Design review of the part built by this model. Coordinates are the model's own, in mm. Face numbers are marked on the shaded views. A direction names the side the tool comes from. Round coordinates to 2 decimals unless told otherwise and drop trailing zeros. Loops run counter-clockwise (first coordinate to the right, second up) from the corner with the lowest first, then second, coordinate; pieces in that order, holes last. Notation, with made-up numbers: (78, 7) -> (115, 7) arc R34 ccw to (115, 37) -> close; hole circle Ø6 at (38.5, 53.5). An arc over 180 degrees is marked (long way). Write each question's results on one line, items separated by ' | '. Start each with the question number.
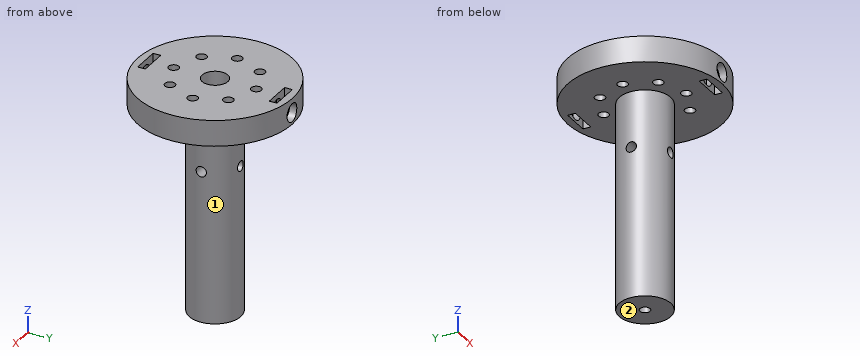
from build123d import *

# Parameters (mm, degrees)
SKETCH1_R               = 30
BOSS_EXTRUDE1_DEPTH     = 10
SKETCH2_R               = 10
BOSS_EXTRUDE2_DEPTH     = 80
SKETCH2_2_R             = 10
BOSS_EXTRUDE3_DEPTH     = 20
SKETCH5_R               = 5
CUT_EXTRUDE1_DEPTH      = 100.498743711
SKETCH6_R               = 2
CUT_EXTRUDE2_DEPTH      = 91.553851381
CIRPATTERN1_COUNT       = 2
CIRPATTERN1_ANGLE       = 90
CUT_EXTRUDE3_DEPTH      = 100.498743801
CUT_EXTRUDE3_DEPTH_BACK = 100.498743801
SKETCH7_R               = 2
SKETCH9_W               = 11
SKETCH9_H               = 3
CUT_EXTRUDE5_DEPTH      = 10
SKETCH10_R              = 3.5
CUT_EXTRUDE6_DEPTH      = 8
SKETCH17_R              = 7.355644599
BOSS_EXTRUDE4_DEPTH     = 25
SKETCH18_R              = 2
CUT_EXTRUDE7_DEPTH      = 10


with BuildPart() as part:
    # Sketch1 → Boss-Extrude1 (new body)
    with BuildSketch(Plane.XY):
        Circle(SKETCH1_R)
    extrude(amount=BOSS_EXTRUDE1_DEPTH)

    # Sketch2 → Boss-Extrude2 (add)
    with BuildSketch(Plane(origin=(0, 0, 0), x_dir=(-1, 0, 0), z_dir=(0, 0, -1))):
        Circle(SKETCH2_R)
    extrude(amount=BOSS_EXTRUDE2_DEPTH)

    # Sketch2_2 → Boss-Extrude3 (add)
    with BuildSketch(Plane(origin=(0, 0, 0), x_dir=(-1, 0, 0), z_dir=(0, 0, -1))):
        Circle(SKETCH2_2_R)
    extrude(amount=BOSS_EXTRUDE3_DEPTH)

    # Sketch5 → Cut-Extrude1 (cut, through all)
    with BuildSketch(Plane(origin=(0, 0, -80), x_dir=(-1, 0, 0), z_dir=(0, 0, -1))):
        Circle(SKETCH5_R)
    extrude(amount=-CUT_EXTRUDE1_DEPTH, mode=Mode.SUBTRACT)

    # Sketch6 → Cut-Extrude2 (cut, symmetric)
    with BuildSketch(Plane(origin=(0, 0, 0), x_dir=(1, 0, 0), z_dir=(0, 1, 0))):
        with Locations(Location((0, 21.5, 0), (0, 0, 270))):
            Circle(SKETCH6_R)
    cut_extrude2 = extrude(amount=CUT_EXTRUDE2_DEPTH, both=True, mode=Mode.SUBTRACT)

    # CirPattern1: Cut-Extrude2 ×2 about axis
    cirpattern1_axis = Axis((0, 0, -80), (0, 0, 1))
    for i in range(1, CIRPATTERN1_COUNT):
        add(cut_extrude2.rotate(cirpattern1_axis, i * CIRPATTERN1_ANGLE / (CIRPATTERN1_COUNT - 1)), mode=Mode.SUBTRACT)

    # Sketch7 → Cut-Extrude3 (cut, two sides: drawn at the far end of the back side and taken through both)
    with BuildSketch(Plane.XY.offset(10).offset(-CUT_EXTRUDE3_DEPTH_BACK)):
        with Locations((0, 16)):
            Circle(SKETCH7_R)
        with Locations((11.313708499, 11.313708499)):
            Circle(SKETCH7_R)
        with Locations((16, 0)):
            Circle(SKETCH7_R)
        with Locations((11.313708499, -11.313708499)):
            Circle(SKETCH7_R)
        with Locations((0, -16)):
            Circle(SKETCH7_R)
        with Locations((-11.313708499, -11.313708499)):
            Circle(SKETCH7_R)
        with Locations((-16, 0)):
            Circle(SKETCH7_R)
        with Locations((-11.313708499, 11.313708499)):
            Circle(SKETCH7_R)
    extrude(amount=CUT_EXTRUDE3_DEPTH + CUT_EXTRUDE3_DEPTH_BACK, mode=Mode.SUBTRACT)

    # Sketch9 → Cut-Extrude5 (cut)
    with BuildSketch(Plane(origin=(0, 0, 0), x_dir=(-1, 0, 0), z_dir=(0, 0, -1))):
        with Locations((0, 25.5)):
            Rectangle(SKETCH9_W, SKETCH9_H)
    cut_extrude5 = extrude(amount=-CUT_EXTRUDE5_DEPTH, mode=Mode.SUBTRACT)

    # Mirror1: Cut-Extrude5 across plane
    add(cut_extrude5.mirror(Plane.ZX), mode=Mode.SUBTRACT)

    # Sketch10 → Cut-Extrude6 (cut)
    with BuildSketch(Plane(origin=(0, -30, 0), x_dir=(-1, 0, 0), z_dir=(0, -1, 0))):
        with Locations(Location((0, -4.5, 0), (0, 0, 90))):
            Circle(SKETCH10_R)
    cut_extrude6 = extrude(amount=-CUT_EXTRUDE6_DEPTH, mode=Mode.SUBTRACT)

    # Mirror2: Cut-Extrude6 across plane
    add(cut_extrude6.mirror(Plane.ZX), mode=Mode.SUBTRACT)

    # Sketch17 → Boss-Extrude4 (add)
    with BuildSketch(Plane(origin=(0, 0, -55), x_dir=(-1, 0, 0), z_dir=(0, 0, -1))):
        Circle(SKETCH17_R)
    extrude(amount=BOSS_EXTRUDE4_DEPTH)

    # Sketch18 → Cut-Extrude7 (cut)
    with BuildSketch(Plane(origin=(0, 0, -80), x_dir=(-1, 0, 0), z_dir=(0, 0, -1))):
        Circle(SKETCH18_R)
    extrude(amount=-CUT_EXTRUDE7_DEPTH, mode=Mode.SUBTRACT)


solid = part.part
1) Insertion check: pin 1 (3 mm diameter, centred on x = 0.5, z = -65.5, fed in from -Y); pin 2 (12 mm diameter, centred on x = 11, z = -40, fed in from -Y); pin 3 (5 mm diameter, centred on x = -11.31, y = 11.31, fed in from -Z). Each pin has a flat end and moves straight along its axis. Give the tip position at first contact, or say it passes through.
2) For the marked faces 1 and 2, list the 3-axis set-ups (+Z, -Z, +X, -X, +Y, -Y) from which the entire face can be reached by the end or side of a thin tool; tool diameter is ignored.
3) Take a section at D-D (x = -6.5). Write out the cut boundary in (y, z), plus the area to 3 significant figures.
4) Take a section at C-C (z = -21.5). Write out the cut boundary in (x, y).
5) Take a section at A-A (y = -16). Write out the cut boundary in (x, z).
6) To check wall thickness, follow line 1 (Y direction, x = 0, z = 3.5); line 2 (Y direction, x = 0, z = -16); line 3 (Z direction, x = 0, y = 23.35). State the ranges of each line that lie inside material, in increasing order. Write a range as from..to.
Geometry check:
1) pin 1: stops at y = -10 | pin 2: stops at y = -8.66 | pin 3: stops at z = 0
2) face 1: -Z | face 2: -Z, +X, -X, +Y, -Y
3) outline: (-29.29, 0) -> (-7.6, 0) -> (-7.6, -80) -> (7.6, -80) -> (7.6, 0) -> (29.29, 0) -> (29.29, 10) -> (-29.29, 10) -> close; hole circle Ø4 at (0, -21.5) | area: 1,790 mm^2
4) outline: (-9.8, -2) arc R10 ccw to (-2, -9.8) -> (-2, -4.58) arc R5 cw to (-4.58, -2) -> close; (-9.8, 2) -> (-4.58, 2) arc R5 cw to (-2, 4.58) -> (-2, 9.8) arc R10 ccw to start; (2, -9.8) arc R10 ccw to (9.8, -2) -> (4.58, -2) arc R5 cw to (2, -4.58) -> close; (2, 4.58) arc R5 cw to (4.58, 2) -> (9.8, 2) arc R10 ccw to (2, 9.8) -> close
5) outline: (-25.38, 0) -> (-2, 0) -> (-2, 10) -> (-25.38, 10) -> close; (2, 0) -> (25.38, 0) -> (25.38, 10) -> (2, 10) -> close
6) line 1: y = -22..-18, -14..-5, 5..14, 18..22 | line 2: y = -10..-5, 5..10 | line 3: z = 0..1, 8..10
